Geometry check sheet. Reference: the model listing, model coordinates, mm. A direction names the side the tool comes from. Round coordinates to 2 decimals unless told otherwise and drop trailing zeros. Write each loop counter-clockwise with the first axis right and the second up, starting at its lowest first coordinate (ties: lowest second). Pieces come first, ordered by that corner, then holes. Notation, with made-up numbers: M -19.75,26 L 5.25,26 A21 ccw 5.25,59 Z; hole C 62,85 d11. An arc over 180 degrees is marked long. Put each result on its own line as item: value. Start each with the question number.
(1) Mould release check, pull along Y, two halves, no side actions. Record for faces 1 (the flat face through (2.5, -2, -18)), 2 (the flat face through (1, 0, -12)), 3 (the cylindrical face through (0.7, -1.4, -3)): pulls with the +Y half, pulls with the -Y half, needs draft (parallel to the pull), parting line crosses it, or undercut.
(2) Section check C-C on z = -1. Record the cut outline in (x, y).
(3) Tool access check on faces 4 (the cylindrical face through (2.7, 2.1, 2.7)), 5 (the flat face through (5.5, -3.44, 0.94)), 6 (the cylindrical face through (1.993, -1.412, -23.002)), 7 (the flat face through (1.5, 1, -25)), 8 (the cylindrical face through (1.268, 0.308, -20.324)). Record the directions out of +Z, -Z, +X, -X, +Y, -Y that give a thin tool (end or side, any length) a straight path to the whole face; none if there is none.
(4) Gauge pin test, flat ends, axial feed: pin 1 (3 mm diameter, centred on x = 1.5, y = 1, fed in from -Z); pin 2 (3 mm diameter, centred on x = 3.5, y = -3, fed in from -Z); pin 3 (0.8 mm diameter, centred on x = 1.5, z = -12.5, fed in from +Y); pin 4 (2.5 mm diameter, centred on y = -1.5, z = 0, fed in from +X). Record the tip position at first contact, or that the pin passes through.
(5) Section check A-A on y = -1.5. Record the cut outline in (x, z), then the cut area to 3 significant figures.
(6) Section check B-B on x = 2.2. Record the cut outline in (y, z), then the cut area to 3 significant figures.
(7) Material ranges on probe 1 along Y at (x, z) = (0.6, -25); probe 2 along Z at (x, y) = (2.7, -1.5); probe 3 along Y at (x, z) = (1.8, -25), recorded low to high.
(8) Section check D-D on x = 3.7. Record the cut outline in (y, z).
from build123d import *

# Parameters (mm, degrees)
SKETCH_1_R               = 4.5
SKETCH_1_W               = 25
SKETCH_1_H               = 6
EXTRUDE_1_DEPTH          = 2.5
EXTRUDE_START            = 2.5
SKETCH_1_5_R             = 4.5
EXTRUDE_3_DEPTH          = 3
CUT_EXTRUDE_2_DEPTH      = 31.602287496
CUT_EXTRUDE_2_DEPTH_BACK = 31.602287496
SKETCH_1_4_R             = 2
FILLET_1_R               = 3
SKETCH_2_R               = 3
CUT_EXTRUDE_3_DEPTH      = 1.5


with BuildPart() as part:
    # 草图1 → 凸台-拉伸1 (new body)
    with BuildSketch(Plane(origin=(0, 0, 0), x_dir=(0, 0, -1), z_dir=(1, 0, 0))):
        with Locations((0, -1.5)):
            Circle(SKETCH_1_R)
        with Locations((25, -1.5)):
            Circle(SKETCH_1_R)
        with Locations((12.5, -3)):
            Rectangle(SKETCH_1_W, SKETCH_1_H)
    extrude(amount=EXTRUDE_1_DEPTH)

    # 草图1<5> → 凸台-拉伸3 (add)
    with BuildSketch(Plane(origin=(0, 0, 0), x_dir=(0, 0, -1), z_dir=(1, 0, 0)).offset(EXTRUDE_START)):
        with Locations(Location((0, -1.5, 0), (0, 0, 270))):
            Circle(SKETCH_1_5_R)
    extrude(amount=EXTRUDE_3_DEPTH)

    # 草图1<4> → 切除-拉伸2 (cut, two sides: drawn at the far end of the back side and taken through both)
    with BuildSketch(Plane(origin=(0, 0, 0), x_dir=(0, 0, -1), z_dir=(1, 0, 0)).offset(-CUT_EXTRUDE_2_DEPTH_BACK)):
        with Locations((0, -1.5)):
            Circle(SKETCH_1_4_R)
        with Locations((25, -1.5)):
            Circle(SKETCH_1_4_R)
    extrude(amount=CUT_EXTRUDE_2_DEPTH + CUT_EXTRUDE_2_DEPTH_BACK, mode=Mode.SUBTRACT)

    # 圆角1
    fillet_1_edges = [part.edges().sort_by_distance(p)[0] for p in [
        (1.25, 0, -20.757359313),
        (1.25, 0, -4.242640687),
    ]]
    fillet(fillet_1_edges, radius=FILLET_1_R)

    # 草图2 → 切除-拉伸3 (cut)
    with BuildSketch(Plane.ZY):
        with Locations((-25, -1.5)):
            Circle(SKETCH_2_R)
        with Locations((0, -1.5)):
            Circle(SKETCH_2_R)
    extrude(amount=-CUT_EXTRUDE_3_DEPTH, mode=Mode.SUBTRACT)


solid = part.part
Answers follow:
1. face 1: needs draft
1. face 2: pulls with the +Y half
1. face 3: undercut
2. outline: M 0,-6 L 2.5,-6 L 2.5,-5.89 L 5.5,-5.89 L 5.5,-3.23 L 1.5,-3.23 L 1.5,-4.33 L 0,-4.33 Z; M 0,1.33 L 1.5,1.33 L 1.5,0.23 L 5.5,0.23 L 5.5,2.89 L 0,2.89 Z
3. face 4: +X
3. face 5: +Z, -Z, +X, +Y, -Y
3. face 6: +X, -X
3. face 7: -X
3. face 8: +X, -X, +Y
4. pin 1: stops at z = -29.39
4. pin 2: stops at z = -29.48
4. pin 3: stops at y = 0
4. pin 4: passes through
5. outline: M 0,-29.5 L 2.5,-29.5 L 2.5,-27 L 1.5,-27 L 1.5,-28 L 0,-28 Z; M 0,-22 L 1.5,-22 L 1.5,-23 L 2.5,-23 L 2.5,-4.5 L 5.5,-4.5 L 5.5,-2 L 1.5,-2 L 1.5,-3 L 0,-3 Z; M 0,3 L 1.5,3 L 1.5,2 L 5.5,2 L 5.5,4.5 L 0,4.5 Z
5. area: 74.0 mm^2
6. outline: M -6,-25 A4.5 ccw long 1.2,-21.4 A3 cw 0,-19 L 0,-6 A3 cw 1.2,-3.6 A4.5 ccw long -6,0 Z; hole C -1.5,-25 d4; hole C -1.5,0 d4
6. area: 208 mm^2
7. probe 1: y = -6 to -4.5, 1.5 to 3
7. probe 2: z = -4.5 to -2, 2 to 4.5
7. probe 3: y = -6 to -3.5, 0.5 to 3
8. outline: C -1.5,0 d9; hole C -1.5,0 d4
